For this review, take the finished solid that the model builds, in its own axes (mm). Round coordinates to 2 decimals unless told otherwise and drop trailing zeros. Write each loop counter-clockwise with the first axis right and the second up, starting at its lowest first coordinate (ties: lowest second). Pieces come first, ordered by that corner, then holes. Notation, with made-up numbers: (-19.75, 22.25) -> (23.25, 22.25) arc R22 ccw to (23.25, 43.25) -> close; hole circle Ø1 at (25.5, -26.5). An arc over 180 degrees is marked (long way). Answer in a Markdown table with one row per item.
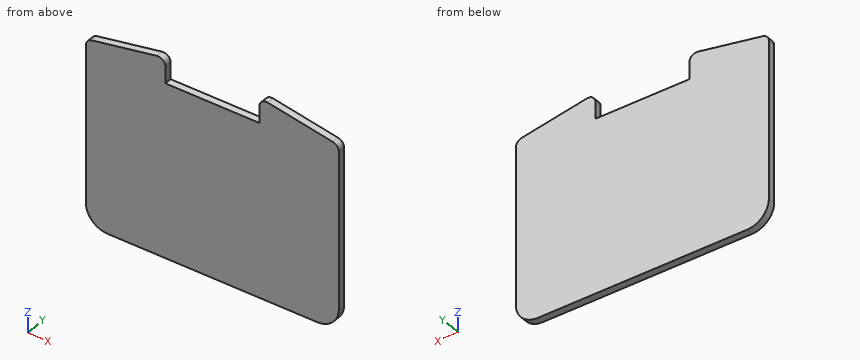
from build123d import *

# Parameters (mm, degrees)
SKETCH_1_W          = 35
SKETCH_1_H          = 25.5
EXTRUDE_1_DEPTH     = 1
EXTRUDE_2_DEPTH     = 1
SKETCH_3_W          = 13
SKETCH_3_H          = 1.5
CUT_EXTRUDE_1_DEPTH = 23.908786524
FILLET_1_R          = 3
FILLET_2_R          = 1


with BuildPart() as part:
    # 草图1 → 凸台-拉伸1 (new body)
    with BuildSketch(Plane(origin=(0, 0, 0), x_dir=(1, 0, 0), z_dir=(0, 1, 0))):
        Rectangle(SKETCH_1_W, SKETCH_1_H)
    extrude(amount=EXTRUDE_1_DEPTH)

    # 草图2 → 凸台-拉伸2 (add)
    with BuildSketch(Plane(origin=(0, 1, 0), x_dir=(1, 0, 0), z_dir=(0, 1, 0))):
        Polygon((-17.5, -12.75), (-6.5, -14.75), (-6.5, -12.75), align=None)
        Polygon((17.5, -12.75), (6.5, -12.75), (6.5, -14.75), align=None)
    extrude(amount=-EXTRUDE_2_DEPTH)

    # 草图3 → 切除-拉伸1 (cut, through all)
    with BuildSketch(Plane(origin=(0, 1, 0), x_dir=(1, 0, 0), z_dir=(0, 1, 0))):
        with Locations((0, -12)):
            Rectangle(SKETCH_3_W, SKETCH_3_H)
    extrude(amount=-CUT_EXTRUDE_1_DEPTH, mode=Mode.SUBTRACT)

    # 圆角1
    fillet_1_edges = [part.edges().sort_by_distance(p)[0] for p in [
        (-17.5, 0.5, -12.75),
        (17.5, 0.5, -12.75),
    ]]
    fillet(fillet_1_edges, radius=FILLET_1_R)

    # 圆角2
    fillet_2_edges = [part.edges().sort_by_distance(p)[0] for p in [
        (-6.5, 0.5, 14.75),
        (6.5, 0.5, 14.75),
        (17.5, 0.5, 12.75),
        (-17.5, 0.5, 12.75),
    ]]
    fillet(fillet_2_edges, radius=FILLET_2_R)


solid = part.part
1) Consider section B-B on x = 2.5. State the section outline as (y, z) points, then the cut area to 3 significant figures.
Solved:
| item | result |
|---|---|
| outline | (0, -12.75) -> (1, -12.75) -> (1, 11.25) -> (0, 11.25) -> close |
| area | 24.0 mm² |
2) For line 1 (Z direction, x = -2, y = 0.7); line 2 (X direction, y = 0.15, z = 12); line 3 (Z direction, x = -12, y = 0.55), list the stretches that pass through material, from the lowest coordinate up. Write a range as [from, to].
Solved:
| item | result |
|---|---|
| line 1 | [-12.75, 11.25] |
| line 2 | [-17.5, -6.5], [6.5, 17.5] |
| line 3 | [-12.75, 13.75] |
3) Consider section A-A on y = 0.65. State the section outline as (x, z) points, then the cut area to 3 significant figures.
Solved:
| item | result |
|---|---|
| outline | (-17.5, -9.75) arc R3 ccw to (-14.5, -12.75) -> (14.5, -12.75) arc R3 ccw to (17.5, -9.75) -> (17.5, 11.92) arc R1 ccw to (16.68, 12.9) -> (7.68, 14.54) arc R1 ccw to (6.5, 13.55) -> (6.5, 11.25) -> (-6.5, 11.25) -> (-6.5, 13.55) arc R1 ccw to (-7.68, 14.54) -> (-16.68, 12.9) arc R1 ccw to (-17.5, 11.92) -> close |
| area | 890 mm² |
4) Consider section C-C on x = -11. State the section outline as (y, z) points, then the cut area to 3 significant figures.
Solved:
| item | result |
|---|---|
| outline | (0, -12.75) -> (1, -12.75) -> (1, 13.93) -> (0, 13.93) -> close |
| area | 26.7 mm² |
5) Clearance check with a flat-ended pin moving along its axis: pin 1 Ø0.5 at (x, y) = (-1.5, 0.5) entering from +Z. State where the tip first meets the part, or that it passes through.
Solved:
| item | result |
|---|---|
| pin 1 | z = 11.25 |
